```python
from build123d import *

# Parameters (mm, degrees)
F0_R     = 3.85
F1_DEPTH = 25
F2_DEPTH = 10
F3_DEPTH = 15


with BuildPart() as f1:
    # F0 (on Top) → F1 (new body)
    with BuildSketch(Plane.XY):
        Circle(F0_R)
    extrude(amount=F1_DEPTH)


with BuildPart() as f1b:
    # F0 (on Top) → F1, piece 2 (new body)
    with BuildSketch(Plane.XY):
        with Locations((0, -18.7460610834)):
            Circle(F0_R)
    extrude(amount=F1_DEPTH)


with BuildPart() as f1c:
    # F0 (on Top) → F1, piece 3 (new body)
    with BuildSketch(Plane.XY):
        with Locations((-22.4686189292, -18.7460610834)):
            Circle(F0_R)
    extrude(amount=F1_DEPTH)

    # F2 (add): a face of the model
    f2_faces = [f1c.faces().sort_by_distance(p)[0] for p in [
        (-22.4686189292, -18.7460610834, 25),
    ]]
    extrude(f2_faces, amount=F2_DEPTH)


with BuildPart() as f1d:
    # F0 (on Top) → F1, piece 4 (new body)
    with BuildSketch(Plane.XY):
        with Locations((-22.4686189292, 0)):
            Circle(F0_R)
    extrude(amount=F1_DEPTH)

    # F3 (add): a face of the model
    f3_faces = [f1d.faces().sort_by_distance(p)[0] for p in [
        (-22.4686189292, 0, 25),
    ]]
    extrude(f3_faces, amount=F3_DEPTH)


solid = f1d.part
```
Here's how the part is built. I have some questions about the finished solid (model axes, mm). Give positions to 0.01 mm unless a question says otherwise; leave off trailing zeros. Loops run counter-clockwise (first coordinate to the right, second up) from the corner with the lowest first, then second, coordinate; pieces in that order, holes last. Notation, with made-up numbers: M 23,33.5 L 33,33.5 A14 ccw 33,56.5 Z; hole C -32.5,0 d2. An arc over 180 degrees is marked long. Return JSON: item names as keys, results as strings.
Item 1: Imagine slicing it at B-B on x = -23.5. List the corners of the cut face in (y, z) for me, then the cut area to 3 significant figures.
A:
{"outline": "M -3.71,0 L 3.71,0 L 3.71,40 L -3.71,40 Z", "area": "297 mm^2"}
Item 2: Please list where these lines run through material, in increasing order: line 1 (X direction, y = -0.25, z = 26.5); line 2 (Y direction, x = -22.25, z = 30.5); line 3 (Y direction, x = -25.5, z = 13.5).
A:
{"line 1": "x = -26.31 to -18.63", "line 2": "y = -3.84 to 3.84", "line 3": "y = -2.37 to 2.37"}
Item 3: I'm going to push flat-ended pins straight in: pin 1 Ø1 at (x, z) = (-25, 31.5) entering from +Y; pin 2 Ø1 at (y, z) = (2.5, 15.5) entering from -X. Where does each tip first touch, or does it pass through?
A:
{"pin 1": "stops at y = 3.27", "pin 2": "stops at x = -25.76"}
Item 4: Imagine slicing it at A-A on z = 35. List the corners of the cut face in (x, y) for me.
A:
{"outline": "C -22.47,0 d7.7"}
Item 5: Imagine slicing it at C-C on y = -1. List the corners of the cut face in (x, z) for me, then the cut area to 3 significant figures.
A:
{"outline": "M -26.19,0 L -18.75,0 L -18.75,40 L -26.19,40 Z", "area": "297 mm^2"}
